Input: part model. Units: mm. Frame: model coordinates. A direction names the side the tool comes from. Round coordinates to 2 decimals unless told otherwise and drop trailing zeros. Loops run counter-clockwise (first coordinate to the right, second up) from the corner with the lowest first, then second, coordinate; pieces in that order, holes last.
1) Section D-D, the plane x = -9. Return loops of the section in (y, z).
2) Section B-B, the plane x = -17. Return loops of the section in (y, z).
3) Ray query, line 1 along X through (y, z) = (10, 2.9); line 2 along X through (y, z) = (10, -1.4); line 3 along X through (y, z) = (26.5, 6.25). Return the intervals inside material, ascending.
4) Section A-A, the plane y = 28. Return loops of the section in (x, z).
5) Section C-C, the plane z = -1.5. Return loops of the section in (x, y).
6) Draft query along Y for faces 1 (the face through (-17, 36, 1)), 2 (the face through (-25, 10, 0.6)), 3 (the face through (-3, 20.5, 6)), 4 (the face through (-29.42, 5.94, -1.97)). Return one class per face: pulls with the +Y half, pulls with the -Y half, needs draft (parallel to the pull), parting line crosses it, or undercut.
7) First-contact query: pin 1 (10 mm diameter, centred on x = -9, y = 10, fed in from +Z); pin 2 (1.2 mm diameter, centred on x = -32, z = 6, fed in from -Y); pin 3 (4 mm diameter, centred on x = -17, y = 28, fed in from -Z); pin 4 (7.5 mm diameter, centred on x = -25, y = 10, fed in from -Z). Flat tips, straight axial feed; report the tip coordinate or a pass-through.
8) Access query for faces 5 (the face through (-31, 20.5, 6)), 6 (the face through (-9, 10, 0)), 7 (the face through (-31, 28, 8)), 8 (the face through (-11.539, 8.053, 2.276)), 9 (the face through (0, 18, 1)). Directions: +Z, -Z, +X, -X, +Y, -Y. A direction counts if a zero-diameter tool reaches every point of the face in a straight line with its end or side. Return the directions, or none.
from build123d import *

# Parameters (mm, degrees)
SKETCH_W      = 34
SKETCH_H      = 36
SKETCH_R      = 3.2
PAD_DEPTH     = 4
SKETCH001_W   = 6.7
SKETCH001_H   = 15.5
PAD001_DEPTH  = 4
FILLET_R      = 5
SKETCH002_R   = 3.2
SKETCH002_R_2 = 6
PAD002_DEPTH  = 4
SKETCH003_R   = 3.2
PAD003_DEPTH  = 0.6
SKETCH004_W   = 20.8
SKETCH004_H   = 19.619243
POCKET_DEPTH  = 4
CHAMFER_SIZE  = 0.4


with BuildPart() as part:
    # Sketch → Pad (new body)
    with BuildSketch(Plane.XY):
        with Locations((-17, 18)):
            Rectangle(SKETCH_W, SKETCH_H)
        with Locations((-17, 28)):
            Circle(SKETCH_R, mode=Mode.SUBTRACT)
        with Locations((-25, 10)):
            Circle(SKETCH_R, mode=Mode.SUBTRACT)
        with Locations((-9, 10)):
            Circle(SKETCH_R, mode=Mode.SUBTRACT)
    extrude(amount=PAD_DEPTH)

    # Sketch001 → Pad001 (new body)
    with BuildSketch(Plane.XY.offset(4)):
        with Locations((-30.65, 28.25)):
            Rectangle(SKETCH001_W, SKETCH001_H)
        with Locations((-3.35, 28.25)):
            Rectangle(SKETCH001_W, SKETCH001_H)
    extrude(amount=PAD001_DEPTH)

    # Fillet
    fillet_edges = [part.edges().sort_by_distance(p)[0] for p in [
        (-34, 0, 2),
        (0, 0, 2),
        (0, 36, 2),
        (0, 36, 6),
        (-34, 36, 6),
        (-34, 36, 2),
    ]]
    fillet(fillet_edges, radius=FILLET_R)

    # Sketch002 → Pad002 (new body)
    with BuildSketch(Plane(origin=(0, 0, 0), x_dir=(1, 0, 0), z_dir=(0, 0, -1))):
        with BuildLine():
            Line((-5, 0), (-29, 0))
            ThreePointArc((-29, 0), (-32.535534, -1.464466), (-34, -5))
            Line((-34, -5), (-34, -31))
            ThreePointArc((-34, -31), (-32.535534, -34.535534), (-29, -36))
            Line((-29, -36), (-5, -36))
            ThreePointArc((-5, -36), (-1.464466, -34.535534), (0, -31))
            Line((0, -31), (0, -5))
            ThreePointArc((0, -5), (-1.464466, -1.464466), (-5, 0))
        make_face()
        with Locations((-17, -28)):
            Circle(SKETCH002_R, mode=Mode.SUBTRACT)
        with Locations((-25, -10)):
            Circle(SKETCH002_R_2, mode=Mode.SUBTRACT)
        with Locations((-9, -10)):
            Circle(SKETCH002_R_2, mode=Mode.SUBTRACT)
    extrude(amount=PAD002_DEPTH)

    # Sketch003 → Pad003 (new body)
    with BuildSketch(Plane(origin=(0, 0, 0), x_dir=(1, 0, 0), z_dir=(0, 0, -1))):
        with Locations((-25, -10)):
            Circle(SKETCH003_R)
        with Locations((-9, -10)):
            Circle(SKETCH003_R)
    extrude(amount=-PAD003_DEPTH)

    # Sketch004 → Pocket (cut)
    with BuildSketch(Plane.XY.offset(4)):
        with Locations((-17, 28.145761)):
            Rectangle(SKETCH004_W, SKETCH004_H)
    extrude(amount=POCKET_DEPTH, mode=Mode.SUBTRACT)

    # Chamfer
    chamfer_edges = [part.edges().sort_by_distance(p)[0] for p in [
        (0, 25.75, 8),
        (-1.464466, 34.535534, 8),
        (-5.8, 36, 8),
        (-28.2, 36, 8),
        (-32.535534, 34.535534, 8),
        (-34, 25.75, 8),
    ]]
    chamfer(chamfer_edges, length=CHAMFER_SIZE)


solid = part.part
Final values:
1. outline: (0, -4) - (4, -4) - (4, 0) - (16, 0) - (16, -4) - (36, -4) - (36, 4) - (13.2, 4) - (13.2, 0.6) - (6.8, 0.6) - (6.8, 4) - (0, 4) - close
2. outline: (0, -4) - (24.8, -4) - (24.8, 4) - (0, 4) - close; (31.2, -4) - (36, -4) - (36, 4) - (31.2, 4) - close
3. line 1: x = -34 to -28.2, -21.8 to -12.2, -5.8 to 0
3. line 2: x = -34 to -31, -19 to -15, -3 to 0
3. line 3: x = -34 to -27.4, -6.6 to 0
4. outline: (-34, -4) - (-20.2, -4) - (-20.2, 4) - (-27.4, 4) - (-27.4, 8) - (-33.6, 8) - (-34, 7.6) - close; (-13.8, -4) - (0, -4) - (0, 7.6) - (-0.4, 8) - (-6.6, 8) - (-6.6, 4) - (-13.8, 4) - close
5. outline: (-34, 5) arc R5 ccw to (-29, 0) - (-5, 0) arc R5 ccw to (0, 5) - (0, 31) arc R5 ccw to (-5, 36) - (-29, 36) arc R5 ccw to (-34, 31) - close; hole circle Ø12 at (-25, 10); hole circle Ø6.4 at (-17, 28); hole circle Ø12 at (-9, 10)
6. face 1: pulls with the +Y half
6. face 2: undercut
6. face 3: pulls with the -Y half
6. face 4: undercut
7. pin 1: stops at z = 4
7. pin 2: stops at y = 20.5
7. pin 3: passes through
7. pin 4: stops at z = 0
8. face 5: +Z, +X, -X, -Y
8. face 6: -Z
8. face 7: +Z, +X, -X, +Y, -Y
8. face 8: +Z
8. face 9: +Z, -Z, +X, +Y, -Y
